Input: dimensioned drawing with shaded views. Units: mm. Origin: part minimum x, y, z. A direction names the side the tool comes from. Give positions to 0.01 mm unless a question says otherwise; leave off trailing zeros. Loops run counter-clockwise (first coordinate to the right, second up) from the corner with the lowest first, then second, coordinate; pieces in that order, holes last.
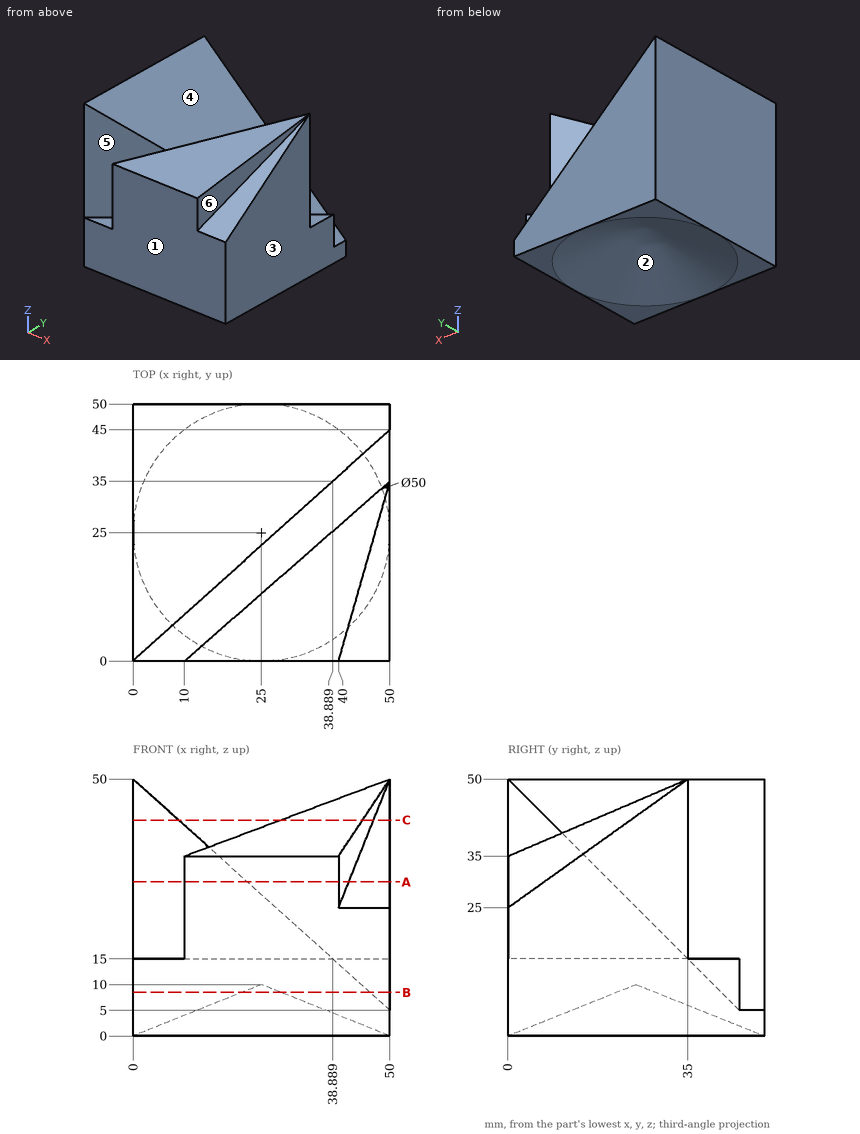
Item 1: Ray query, probe 1 along Y at (x, z) = (17.5, 31.5); probe 2 along Y at (x, z) = (27.5, 24.5); probe 3 along Z at (x, y) = (24, 12.5). Return the intervals inside material, ascending.
Values follow:
probe 1: y = 0 to 6.56, 15.75 to 50
probe 2: y = 0 to 15.31, 24.75 to 50
probe 3: z = 4.98 to 15
Item 2: Section query C-C on z = 42. Return loops of the section in (x, y), plus the area to 3 significant figures.
Values follow:
outline: (0, 0) - (8.89, 8) - (8.89, 50) - (0, 50) - close; (28.67, 16.33) - (44.67, 16.33) - (46.8, 23.8) - (50, 23.8) - (50, 35) - close
area: 576 mm2
Item 3: Set-up query: the marked faces 4, 5 and 6. Return all of +Z, -Z, +X, -X, +Y, -Y with unobstructed straight access to the full face (end or side cutting, diameter ignored); none if empty.
Values follow:
face 4: +Z, +Y
face 5: +Z
face 6: +Z, +X, -Y
Item 4: Pin query (flat end, axial travel): pin 1 (12 mm diameter, centred on x = 29.5, z = 32.5, fed in from +Y); pin 2 (6 mm diameter, centred on x = 35, y = 32, fed in from +Z); pin 3 (22.5 mm diameter, centred on x = 16.5, y = 18, fed in from +Z) (3 decimals). Return the tip coordinate at first contact, or that it passes through.
Values follow:
pin 1: stops at y = 22.31
pin 2: stops at z = 21.2
pin 3: stops at z = 45.275
Item 5: Section query B-B on z = 8.5. Return loops of the section in (x, y).
Values follow:
outline: (0, 0) - (50, 0) - (50, 45) - (46.11, 41.5) - (46.11, 50) - (0, 50) - close; hole circle Ø7.5 at (25, 25)
Item 6: Draft query along X for the marked faces 1, 2 and 3. Return one class per face: +X half, -X half, draft (parallel to the pull), parting line (faces both ways), or undercut.
Values follow:
face 1: draft
face 2: undercut
face 3: +X half
Item 7: Section query A-A on z = 30. Return loops of the section in (x, y).
Values follow:
outline: (0, 0) - (22.22, 20) - (22.22, 50) - (0, 50) - close; (10, 0) - (40, 0) - (42, 7) - (50, 7) - (50, 35) - close
